Autodesk Inventor part; units mm, degrees
ref_plane "Work Plane1" through (1.525, 0, 0) normal (0, 0, 1) x (1, 0, 0)
ref_plane "YZ Plane" through (0, 0, 0) normal (1, 0, 0) x (0, 1, 0)
ref_plane "XZ Plane" through (0, 0, 0) normal (0, 1, 0) x (-1, 0, 0)
sketch "Sketch1" plane through (0, 0, 0) normal (0, 0, 1) x (1, 0, 0)
  line L0 (0, 7.315) -> (0, 5)
  line L1 (4.5, 5) -> (40, 5)
  line L2 (40, 5) -> (40, 0)
  line L3 (40, 0) -> (-0.6001, 0)
  line L4 (-8.7201, 0) -> (48.12, 0)
  line L5 (-0.6001, 0) -> (-0.6001, 7.315)
  line L6 (-0.6001, 7.315) -> (0, 7.315)
  line L7 (4.5, 5) -> (3.5797, 5)
  line L8 (3.5797, 5) -> (0, 5)
  line L9 (0, -1.463) -> (0, 8.778)
  dimension "d0" = 40
  dimension "d1" = 35.5
  dimension "d2" = 10
  dimension "d9" = 0.6001
  dimension "d10" = 14.63
  dimension "d13" = 0.9203
  dimension "d14" = 10
revolve "Body" add sketch "Sketch1" angle 360 about axis through (40, 0, 0) along (-1, 0, 0)
sketch "Sketch2" plane through (-0.6001, 0, 0) normal (-1, 0, 0) x (0, 0, 1)
  line L0 (0, 9.2376) -> (8, 4.6188)
  line L1 (8, 4.6188) -> (8, -4.6188)
  line L2 (8, -4.6188) -> (0, -9.2376)
  line L3 (0, -9.2376) -> (-8, -4.6188)
  line L4 (-8, -4.6188) -> (-8, 4.6188)
  line L5 (-8, 4.6188) -> (0, 9.2376)
  point P0 (0, 0)
  point P1 (0, 0)
  dimension "d11" = 16
extrude "Head" add sketch "Sketch2" along normal blind 5.8
sketch "Sketch4" plane through (0, 0, 0) normal (0, 0, 1) x (1, 0, 0)
  line L0 (-6.4001, 8) -> (-6.4001, 9.2376)
  line L1 (-6.4001, 9.2376) -> (-5.6856, 9.2376)
  line L2 (-5.6856, 9.2376) -> (-6.4001, 8)
  line L3 (-7.5601, 0) -> (0.5599, 0)
  line L4 (-0.6001, 9.2376) -> (-6.4001, 9.2376)
  line L5 (-6.4001, 4.6188) -> (-6.4001, 9.2376)
  dimension "d5" = 30
  dimension "d19" = 16
revolve "Chamfer1" cut sketch "Sketch4" angle 360 about axis through (-10, 0, 0) along (1, 0, 0)
thread "Thread"
chamfer "Chamfer2" distance 0.9202 distance2 0.9203 1 edges at (40, -5, 0) measured on face at (40, 1.2281, 0.495)
ref_plane "Work Plane1" through (1.525, 0, 0) normal (0, 0, 1) x (1, 0, 0)
equation "\"d11\" = SW"
equation "\"d3\" = KOH - SD"
equation "\"d15\" = GEL"
equation "\"d6\" = -0.5 * SPD + 0.5 * GD"
equation "\"d0\" = NLG"
equation "\"d1\" = GEL"
equation "\"d2\" = GD"
equation "\"d10\" = SD2"
equation "\"d14\" = BDM"
equation "\"d5\" = ANG1"
equation "\"d19\" = SW0"
equation "\"NLG\" = 40"
equation "\"GD\" = NND"
equation "\"BDM\" = NND"
equation "\"KOH\" = 6.4"
equation "\"GEL\" = 35.5"
equation "\"SW\" = 16"
equation "\"SW0\" = SW"
equation "\"SPD\" = NND - 1.2269 * PTC"
equation "\"SD2\" = 14.63"
equation "\"SD\" = 0.6"
equation "\"ANG1\" = 30deg"
equation "\"GAL\" = 0.61345 * PTC"
equation "\"GUL\" = 0.61345 * PTC"
equation "\"RR\" = 0.4"
equation "\"GD1\" = THREADDIA - 1.2269 * PTC"
equation "\"SDH\" = SD2"
equation "\"SDHG\" = 4.5"
equation "\"TOA\" = 30deg"
equation "\"PTC\" = 1.5"
equation "\"E0\" = 18.48"
properties part number "ISO 4017 - M10 x 40" material "Stainless Steel, 440C"
Check sheet for the modelled part. Datum: model origin and axes. Units: mm. A direction names the side the tool comes from. Round coordinates to 2 decimals unless told otherwise and drop trailing zeros. Loops run counter-clockwise (first coordinate to the right, second up) from the corner with the lowest first, then second, coordinate; pieces in that order, holes last. Notation, with made-up numbers: (-1.75, 32.25) -> (42.25, 32.25) arc R21 cw to (42.25, 61.25) -> close; hole circle Ø11 at (67.5, 34.5). An arc over 180 degrees is marked (long way). Write item = value, one per line. Start each with the question number.
1) Thickness scan on probe 1 along X at (y, z) = (-1.75, -7); probe 2 along Y at (x, z) = (30, 0.25); probe 3 along X at (y, z) = (7.5, -2.75). Record the ranges inside material, lowest first.
2) Sectioned sample at A-A, the plane x = 31. Record the cut outline in (y, z), plus the area to 3 significant figures.
3) Set-up check for faces 1 (the conical face through (-6.226, -4.168, -7.179)), 2 (the cylindrical face through (19.27, -1.08, 4.88)): record each of +Z, -Z, +X, -X, +Y, -Y from which the full face is reachable in a straight line by a thin tool's end or side.
4) Gauge pin test, flat ends, axial feed: pin 1 Ø5 at (y, z) = (5.5, 2.5) entering from +X; pin 2 Ø1.5 at (y, z) = (7.5, 1.5) entering from +X; pin 3 Ø2 at (x, y) = (11, -0.5) entering from -Z; pin 4 Ø2 at (x, z) = (14, -2.5) entering from +Y. Record the tip position at first contact, or that the pin passes through.
Results are:
q1.probe_1 = -6.4 to 0
q1.probe_2 = -4.99 to 4.99
q1.probe_3 = -6.4 to -0.6
q2.outline = circle Ø10 at (0, 0)
q2.area = 78.5 mm^2
q3.face_1 = -Z, -X, -Y
q3.face_2 = +X
q4.pin_1 = 40
q4.pin_2 = 0
q4.pin_3 = -5
q4.pin_4 = 4.77
